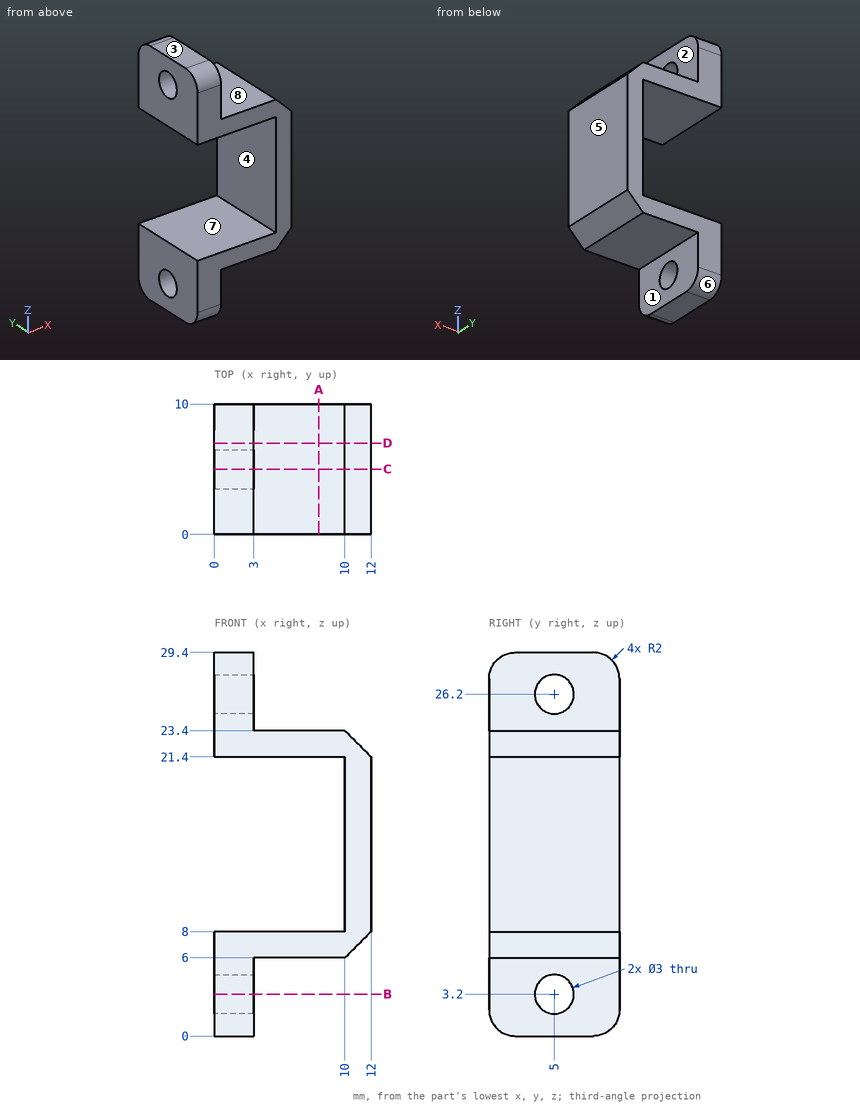
Study the drawing (mm; zero at the part's minimum x, y, z) and answer. A direction names the side the tool comes from. Give positions to 0.01 mm unless a question says otherwise; leave off trailing zeros. Write each loop counter-clockwise with the first axis right and the second up, starting at its lowest first coordinate (ties: lowest second). Pieces come first, ordered by that corner, then holes. Notation, with made-up numbers: (-36.5, 21) -> (12.5, 21) arc R25 cw to (12.5, 34) -> close; hole circle Ø2 at (59.5, 85.25). An arc over 180 degrees is marked (long way). Write item = value, one per line. Start each with the question number.
1) The part is cut by section B-B, the plane z = 3.2. Determine the outline of the cut face in (x, y), and give its area (3 significant figures).
2) Determine the mould class of the marked faces 5, 6, 7 and 8 for opening direction Z: +Z half, -Z half, draft (parallel to the pull), parting line (faces both ways), or undercut.
3) Each of these flat-tipped pins is pushed along its axis until it touches: pin 1 (1.8 mm diameter, centred on y = 5, z = 3.2, fed in from +X); pin 2 (3 mm diameter, centred on y = 5.5, z = 25, fed in from +X); pin 3 (2 mm diameter, centred on x = 6.5, y = 7, fed in from -Z). Where does it stop, or does it pass through?
4) The part is cut by section D-D, the plane y = 7. Determine the outline of the cut face in (x, z).
5) The part is cut by section A-A, the plane x = 8. Determine the outline of the cut face in (y, z).
6) Straight lines are drawn through the part: line 1 along Z through (x, y) = (6, 5.75); line 2 along Y through (x, z) = (0.9, 3.2); line 3 along X through (y, z) = (6.25, 16.5). For each, find the intervals that lie inside material, in ascending order.
7) The part is cut by section C-C, the plane y = 5. Determine the outline of the cut face in (x, z).
8) Which of the six approach directions +Z, -Z, +X, -X, +Y, -Y give full straight-line access (tool end or side, diameter ignored) to the marked faces 1, 2, 3 and 4?
Solutions:
q1.outline = (0, 0) -> (3, 0) -> (3, 3.5) -> (0, 3.5) -> close; (0, 6.5) -> (3, 6.5) -> (3, 10) -> (0, 10) -> close
q1.area = 21.0 mm²
q2.face_5 = draft
q2.face_6 = -Z half
q2.face_7 = undercut
q2.face_8 = +Z half
q3.pin_1 = through
q3.pin_2 = 3
q3.pin_3 = 6
q4.outline = (0, 0) -> (3, 0) -> (3, 6) -> (10, 6) -> (12, 8) -> (12, 21.4) -> (10, 23.4) -> (3, 23.4) -> (3, 29.4) -> (0, 29.4) -> (0, 21.4) -> (10, 21.4) -> (10, 8) -> (0, 8) -> close
q5.outline = (0, 6) -> (10, 6) -> (10, 8) -> (0, 8) -> close; (0, 21.4) -> (10, 21.4) -> (10, 23.4) -> (0, 23.4) -> close
q6.line_1 = 6 to 8, 21.4 to 23.4
q6.line_2 = 0 to 3.5, 6.5 to 10
q6.line_3 = 10 to 12
q7.outline = (0, 0) -> (3, 0) -> (3, 1.7) -> (0, 1.7) -> close; (0, 4.7) -> (3, 4.7) -> (3, 6) -> (10, 6) -> (12, 8) -> (12, 21.4) -> (10, 23.4) -> (3, 23.4) -> (3, 24.7) -> (0, 24.7) -> (0, 21.4) -> (10, 21.4) -> (10, 8) -> (0, 8) -> close; (0, 27.7) -> (3, 27.7) -> (3, 29.4) -> (0, 29.4) -> close
q8.face_1 = -Z, +X, +Y, -Y
q8.face_2 = +Z, +X, +Y, -Y
q8.face_3 = +Z, +X, -X, +Y, -Y
q8.face_4 = -X, +Y, -Y
